The listing builds one solid part. Answer for the finished solid, in the listing's coordinates (mm). A direction names the side the tool comes from. Give positions to 0.01 mm unless a question says otherwise; leave off trailing zeros. Order: outer loops, then holes, each group sorted by start corner. A loop starts at its lowest first (then second) coordinate and runs counter-clockwise, first axis right, second up. Notation, with made-up numbers: (-38, 85) - (-22, 85) arc R29 ccw to (-22, 123) - close; hole circle Ø11 at (-32, 4). An arc over 180 degrees is marked (long way). Answer in a Markdown table with one row per item.
Autodesk Inventor part; units mm, degrees
ref_plane "YZ Plane" through (0, 0, 0) normal (1, 0, 0) x (0, 1, 0)
ref_plane "XZ Plane" through (0, 0, 0) normal (0, 1, 0) x (-1, 0, 0)
ref_plane "XY Plane" through (0, 0, 0) normal (0, 0, 1) x (1, 0, 0)
sketch "Sketch1" plane through (0, 0, 0) normal (0, 0, 1) x (1, 0, 0)
  line L0 (-40, -29) -> (-40, 29)
  line L1 (-40, 29) -> (40, 29)
  line L2 (40, 29) -> (40, -29)
  line L3 (40, -29) -> (-40, -29)
  line L4 (-40, -29) -> (40, 29) construction
  line L5 (-40, 29) -> (40, -29) construction
  line L6 (40, 17.5) -> (70, 17.5)
  line L7 (70, 17.5) -> (70, -17.5)
  line L8 (70, -17.5) -> (40, -17.5)
  line L9 (40, -17.5) -> (40, 17.5)
  point P0 (0, 0)
  dimension "d0" = 58
  dimension "d1" = 80
  dimension "d2" = 30
  dimension "d3" = 35
sketch "Sketch2" plane through (0, 0, 0) normal (0, 0, 1) x (1, 0, 0)
  point P0 (0, 0)
extrude "Extrusion1" add sketch "Sketch1" along normal blind 5
sketch "Sketch3" plane through (0, 0, 5) normal (0, 0, 1) x (1, 0, 0)
  line L0 (-19, 26.9) -> (19, 26.9)
  line L1 (19, 26.9) -> (19, 23.9)
  line L2 (19, 23.9) -> (-19, 23.9)
  line L3 (-19, 23.9) -> (-19, 26.9)
  line L4 (-19, -23.9) -> (19, -23.9)
  line L5 (19, -23.9) -> (19, -26.9)
  line L6 (19, -26.9) -> (-19, -26.9)
  line L7 (-19, -26.9) -> (-19, -23.9)
  line L8 (61.9, 14.9) -> (64.9, 14.9)
  line L9 (64.9, 14.9) -> (64.9, -14.9)
  line L10 (64.9, -14.9) -> (61.9, -14.9)
  line L11 (61.9, -14.9) -> (61.9, 14.9)
  line L12 (40, 29) -> (-40, 29)
  line L13 (-40, 29) -> (-40, -29)
  line L14 (40, 17.5) -> (40, 29)
  line L15 (-40, -29) -> (40, -29)
  line L16 (40, -29) -> (40, -17.5)
  line L17 (70, -17.5) -> (70, 17.5)
  line L18 (70, 17.5) -> (40, 17.5)
  line L19 (40, -17.5) -> (70, -17.5)
  point P0 (0, 0)
  dimension "d6" = 2.1
  dimension "d7" = 3
  dimension "d8" = 21
  dimension "d9" = 21
  dimension "d10" = 2.1
  dimension "d11" = 21
  dimension "d12" = 21
  dimension "d13" = 3
  dimension "d14" = 5.1
  dimension "d15" = 2.6
  dimension "d16" = 2.6
  dimension "d17" = 3
extrude "Extrusion2" add sketch "Sketch3" along normal blind 2 contours L0 L1 L2 L3 | L4 L5 L6 L7 | L8 L9 L10 L11
properties part number "CageV5 Lid"
Item 1: Which of the six approach directions +Z, -Z, +X, -X, +Y, -Y give full straight-line access (tool end or side, diameter ignored) to faces 5 (the face through (63, 14.9, 6)), 6 (the face through (63, -14.9, 6)), 7 (the face through (19, 25, 6))?
Answer block:
| item | result |
|---|---|
| face 5 | +Z, +X, -X, +Y |
| face 6 | +Z, +X, -X, -Y |
| face 7 | +Z, +X, +Y, -Y |
Item 2: Consider line 1 (X direction, y = 7, z = 5.5); line 2 (Z direction, x = -0.5, y = -5); line 3 (Y direction, x = 54, z = 1). Determine where each line is inside the solid, lowest interval first.
Answer block:
| item | result |
|---|---|
| line 1 | 61.9 to 64.9 |
| line 2 | 0 to 5 |
| line 3 | -17.5 to 17.5 |
Item 3: Determine the mould class of faces 1 (the face through (0, -23.9, 6)), 2 (the face through (0, -26.9, 6)), 3 (the face through (0, 26.9, 6)), 4 (the face through (2, 0, 5)) for opening direction Y: pulls with the +Y half, pulls with the -Y half, needs draft (parallel to the pull), parting line crosses it, or undercut.
Answer block:
| item | result |
|---|---|
| face 1 | undercut |
| face 2 | pulls with the -Y half |
| face 3 | pulls with the +Y half |
| face 4 | undercut |
Item 4: Each of these flat-tipped pins is pushed along its axis until it touches: P1, Ø0.6, axis at x = -7.5, z = 6, coming from the +Y side; P2, Ø5, axis at x = 13, y = -9, coming from the -Z side; P3, Ø8, axis at x = 33.5, y = 9.5, coming from the +Z side; P4, Ø1, axis at y = -1.5, z = 6, coming from the -X side. Where does it stop, or does it pass through?
Answer block:
| item | result |
|---|---|
| P1 | y = 26.9 |
| P2 | z = 0 |
| P3 | z = 5 |
| P4 | x = 61.9 |
Item 5: Find section A-A on y = 8.5. Write down the section's boundary in (x, z).
Answer block:
| item | result |
|---|---|
| outline | (-40, 0) - (70, 0) - (70, 5) - (64.9, 5) - (64.9, 7) - (61.9, 7) - (61.9, 5) - (-40, 5) - close |
Item 6: Find section D-D on y = 21. Write down the section's boundary in (x, z), then the cut area to 3 significant figures.
Answer block:
| item | result |
|---|---|
| outline | (-40, 0) - (40, 0) - (40, 5) - (-40, 5) - close |
| area | 400 mm² |
Item 7: Find section C-C on x = -8.5. Write down the section's boundary in (y, z), then the cut area to 3 significant figures.
Answer block:
| item | result |
|---|---|
| outline | (-29, 0) - (29, 0) - (29, 5) - (26.9, 5) - (26.9, 7) - (23.9, 7) - (23.9, 5) - (-23.9, 5) - (-23.9, 7) - (-26.9, 7) - (-26.9, 5) - (-29, 5) - close |
| area | 302 mm² |
Item 8: Find section B-B on z = 2. Write down the section's boundary in (x, y).
Answer block:
| item | result |
|---|---|
| outline | (-40, -29) - (40, -29) - (40, -17.5) - (70, -17.5) - (70, 17.5) - (40, 17.5) - (40, 29) - (-40, 29) - close |
